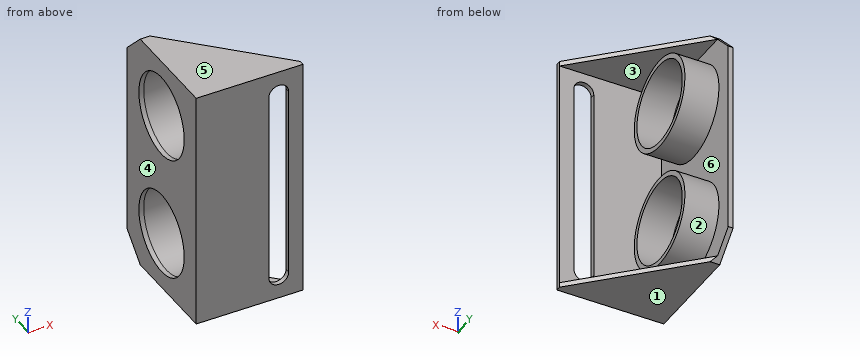
Autodesk Inventor part; units mm, degrees
ref_plane "YZ Plane" through (0, 0, 0) normal (1, 0, 0) x (0, 1, 0)
ref_plane "XZ Plane" through (0, 0, 0) normal (0, 1, 0) x (-1, 0, 0)
ref_plane "XY Plane" through (0, 0, 0) normal (0, 0, 1) x (1, 0, 0)
sketch "Sketch1" plane through (0, 0, 0) normal (0, 1, 0) x (-1, 0, 0)
  line L0 (-11, 25) -> (-11, -25)
  line L1 (-11, -25) -> (11, -25)
  line L2 (11, -25) -> (11, 25)
  line L3 (11, 25) -> (-11, 25)
  line L4 (-11, 25) -> (11, -25) construction
  line L5 (-11, -25) -> (11, 25) construction
  line L6 (11, 25) -> (10, 25)
  line L7 (10, 25) -> (10, -25)
  line L8 (11, 25) -> (11, 24)
  line L9 (11, 24) -> (-11, 24)
  line L10 (11, -25) -> (11, -24)
  line L11 (11, -24) -> (-11, -24)
  point P0 (0, 0)
  dimension "d0" = 50
  dimension "d1" = 22
  dimension "d2" = 1
  dimension "d3" = 1
  dimension "d4" = 1
extrude "Extrusion1" add sketch "Sketch1" along normal blind 1
sketch "Sketch2" plane through (0, 1, 0) normal (0, 1, 0) x (1, 0, 0)
  line L0 (11, -25) -> (11, 25)
  line L1 (-11, -25) -> (11, -25)
  line L2 (11, -25) -> (-11, -25)
  line L3 (-11, -25) -> (-11, -24)
  line L4 (-11, 25) -> (-11, -25)
  line L5 (-11, -24) -> (11, -24)
  line L6 (-11, -25) -> (-10, -25)
  line L7 (-10, -25) -> (-10, 25)
  line L8 (11, 25) -> (-11, 25)
  line L9 (-11, 25) -> (-11, 24)
  line L10 (-11, 24) -> (11, 24)
  point P0 (0, 0)
  dimension "d7" = 1
  dimension "d8" = 1
  dimension "d9" = 1
extrude "Extrusion2" add sketch "Sketch2" along normal blind 25 contours L1 L3 L5 L7 | L5 L4 L10 L7 | L10 L4 L8 L7
extrude "Extrusion3" add sketch "Sketch2" along normal blind 25 contours L1 L7 L5 L0 | L1 L3 L5 L7 | L10 L7 L8 L0 | L10 L4 L8 L7
sketch "Sketch3" plane through (-11, 0, 25) normal (0, 0, 1) x (1, 0, 0)
  point P0 (11, 0)
sketch "Sketch4" plane through (-11, 0, -25) normal (-1, 0, 0) x (0, 0, 1)
  line L0 (49, 26) -> (1, 26)
  line L1 (25, 26) -> (45, 26)
  line L2 (25, 26) -> (5, 26)
  line L3 (50, 0) -> (50, 26)
  line L4 (50, 26) -> (50, 21)
  line L5 (50, 21) -> (45, 26)
  line L6 (0, 0) -> (0, 26)
  line L7 (0, 26) -> (0, 21)
  line L8 (0, 21) -> (5, 26)
  line L9 (50, 26) -> (45, 26)
  line L10 (0, 26) -> (5, 26)
  line L11 (0, 26) -> (50, 26)
  point P0 (25, 0)
  dimension "d14" = 20
  dimension "d15" = 20
  dimension "d16" = 5
  dimension "d17" = 5
extrude "Extrusion4" cut sketch "Sketch4" against normal blind 25
sketch "Sketch5" plane through (-11, 0, 25) normal (0, 0, 1) x (1, 0, 0)
  line L0 (1, 22) -> (1, 26)
  line L1 (1, 22) -> (22, 1)
  line L2 (22, 22) -> (1, 22)
  line L3 (1, 22) -> (22, 22)
  line L4 (22, 22) -> (22, 1)
  point P0 (11, 0)
extrude "Extrusion5" cut sketch "Sketch5" against normal through all
sketch "Sketch6" plane through (-10, 1, 24) normal (1, 0, 0) x (0, 0, -1)
  line L0 (4, 25) -> (44, 25)
  line L1 (24, 25) -> (24, -1) construction
  line L2 (0, 21) -> (0, 0) construction
  line L3 (0, 12) -> (48, 12) construction
  line L4 (48, 0) -> (48, 21) construction
  line L5 (24, 12) -> (20.5, 12) construction
  line L6 (20.5, 12) -> (27.5, 12) construction
  line L7 (20.5, 12) -> (1.5, 12) construction
  circle A0 centre (11, 12) radius 9.5
  circle A1 centre (11, 12) radius 8.5
  dimension "d22" = 3.5
  dimension "d23" = 7
  dimension "d24" = 19
  dimension "d25" = 1
extrude "Extrusion6" add sketch "Sketch6" along normal blind 7
extrude "Extrusion7" cut sketch "Sketch6" against normal blind 7 contours A1
ref_plane "Work Plane1" through (-11, 0, 0) normal (0, 0, 1) x (1, 0, 0)
mirror "Mirror1" about plane through (-11, 0, 0) normal (0, 0, 1) of "Extrusion6"
mirror "Mirror2" about plane through (-11, 0, 0) normal (0, 0, 1) of "Extrusion6"
sketch "Sketch7" plane through (-10, 13, -13) normal (1, 0, 0) x (0, 0, -1)
  circle A0 centre (0, 0) radius 8.5
  point P0 (-13, -13)
extrude "Extrusion8" cut sketch "Sketch7" against normal blind 7
sketch "Sketch8" plane through (0, 1, 0) normal (0, 1, 0) x (1, 0, 0)
  line L0 (-10, -24) -> (11, -24)
  line L1 (11, -24) -> (6, -24)
  line L2 (6, -24) -> (6, -20) construction
  line L3 (11, 24) -> (-10, 24) construction
  line L4 (11, 24) -> (6, 24) construction
  line L5 (6, 24) -> (6, 20) construction
  line L6 (6, 20) -> (6, -20) construction
  line L7 (8.0416, 20) -> (8.0416, -20)
  line L8 (3.9584, -20) -> (3.9584, 20)
  arc A0 (8.0416, 20) -> (3.9584, 20) centre (6, 20) ccw
  arc A1 (3.9584, -20) -> (8.0416, -20) centre (6, -20) ccw
  point P0 (0, 0)
  point P1 (6, 0)
  dimension "d32" = 5
  dimension "d33" = 4
  dimension "d34" = 5
  dimension "d35" = 4
extrude "Extrusion9" cut sketch "Sketch8" against normal blind 7
properties part number "Ultra Sonic Sensor Mounting"
Geometry: final body of the model. Coordinates: model frame, mm. Face numbers are marked on the shaded views. A direction names the side the tool comes from. Round coordinates to 2 decimals unless told otherwise and drop trailing zeros. Write each loop counter-clockwise with the first axis right and the second up, starting at its lowest first coordinate (ties: lowest second). Pieces come first, ordered by that corner, then holes. Notation, with made-up numbers: (70, 79) -> (95, 79) arc R15 ccw to (95, 98) -> close; hole circle Ø11 at (-14, 22.25). An arc over 180 degrees is marked (long way). Return JSON: item names as keys, results as strings.
Q1. Section C-C on z = 13. Return the cut outline in (x, y).
From the geometry:
{"outline": "(-11, 0) -> (3.96, 0) -> (3.96, 1) -> (-10, 1) -> (-10, 3.5) -> (-3, 3.5) -> (-3, 4.5) -> (-11, 4.5) -> close; (-11, 21.5) -> (-3, 21.5) -> (-3, 22.5) -> (-10, 22.5) -> (-10, 26) -> (-11, 26) -> close; (8.04, 0) -> (11, 0) -> (11, 1) -> (8.04, 1) -> close"}
Q2. Section D-D on x = 4.75. Return the cut outline in (y, z).
From the geometry:
{"outline": "(0, -25) -> (7.25, -25) -> (7.25, -24) -> (1, -24) -> (1, -21.61) -> (0, -21.61) -> close; (0, 21.61) -> (1, 21.61) -> (1, 24) -> (7.25, 24) -> (7.25, 25) -> (0, 25) -> close"}
Q3. Mould query, pull axis Z, two halves, no side actions, for the marked faces 3, 4, 5 and 6. Classes: +Z half, -Z half, draft (parallel to the pull), parting line (faces both ways), or undercut.
From the geometry:
{"face 3": "undercut", "face 4": "draft", "face 5": "+Z half", "face 6": "undercut"}
Q4. Ray query, line 1 (Y direction, x = -5, z = 19.5); line 2 (Y direction, x = -5.5, z = 13); line 3 (Z direction, x = -9.5, y = 6). Return the intervals inside material, ascending.
From the geometry:
{"line 1": "0 to 1, 6.07 to 7.52, 18.48 to 19.93", "line 2": "0 to 1, 3.5 to 4.5, 21.5 to 22.5", "line 3": "-25 to -24, -19.42 to -17.82, -8.18 to -6.58, 6.58 to 8.18, 17.82 to 19.42, 24 to 25"}
Q5. Set-up query: the marked faces 1 and 2. Return all of +Z, -Z, +X, -X, +Y, -Y with unobstructed straight access to the full face (end or side cutting, diameter ignored); none if empty.
From the geometry:
{"face 1": "-Z, +X, -X, +Y, -Y", "face 2": "+X"}
Q6. Section B-B on x = -8.5. Return the cut outline in (y, z).
From the geometry:
{"outline": "(0, -25) -> (20.5, -25) -> (20.5, -24) -> (1, -24) -> (1, 24) -> (20.5, 24) -> (20.5, 25) -> (0, 25) -> close; circle Ø19 at (13, -13); circle Ø19 at (13, 13); hole circle Ø17 at (13, -13); hole circle Ø17 at (13, 13)"}
Q7. First-contact query: pin 1 Ø2 at (x, z) = (0.5, -19) entering from +Y; pin 2 Ø12 at (y, z) = (21.5, 0.5) entering from +X; pin 3 Ø3 at (x, z) = (0.5, -12) entering from -Y. Flat tips, straight axial feed; report the tip coordinate or a pass-through.
From the geometry:
{"pin 1": "y = 1", "pin 2": "x = -3", "pin 3": "y = 0"}
Q8. Section A-A on y = 13. Return the cut outline in (x, z), and give its area (3 significant figures).
From the geometry:
{"outline": "(-11, -25) -> (-1, -25) -> (-1, -24) -> (-10, -24) -> (-10, -22.5) -> (-3, -22.5) -> (-3, -21.5) -> (-11, -21.5) -> close; (-11, -4.5) -> (-3, -4.5) -> (-3, -3.5) -> (-10, -3.5) -> (-10, 3.5) -> (-3, 3.5) -> (-3, 4.5) -> (-11, 4.5) -> close; (-11, 21.5) -> (-3, 21.5) -> (-3, 22.5) -> (-10, 22.5) -> (-10, 24) -> (-1, 24) -> (-1, 25) -> (-11, 25) -> close", "area": "62.0 mm2"}
